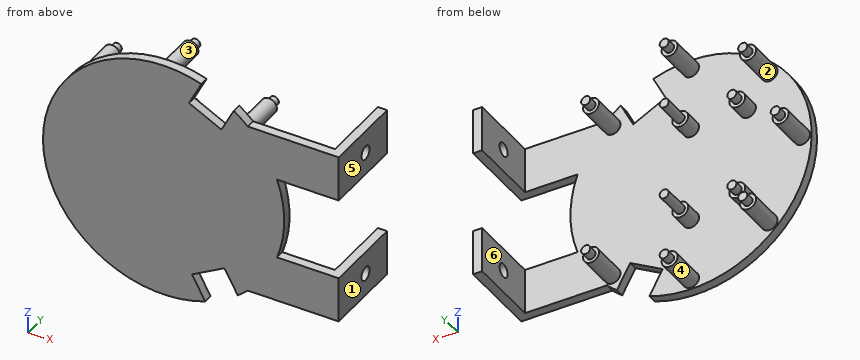
Autodesk Inventor part; units mm, degrees
ref_plane "YZ Plane" through (0, 0, 0) normal (1, 0, 0) x (0, 1, 0)
ref_plane "XZ Plane" through (0, 0, 0) normal (0, 1, 0) x (-1, 0, 0)
ref_plane "XY Plane" through (0, 0, 0) normal (0, 0, 1) x (1, 0, 0)
sketch "Teller" plane through (0, 0, 0) normal (0, 1, 0) x (-1, 0, 0)
  line L0 (-16.2935, -20.8991) -> (-13.3783, -15.6549)
  line L1 (-13.3783, -15.6549) -> (-6.2348, -19.626)
  line L2 (-6.2348, -19.626) -> (-9.15, -24.8702)
  line L3 (-8.2927, 25.1691) -> (-5.5764, 19.8191)
  line L4 (-5.5764, 19.8191) -> (-12.7097, 16.1974)
  line L5 (-12.7097, 16.1974) -> (-15.426, 21.5474)
  arc A0 (-9.15, -24.8702) -> (-8.2927, 25.1691) centre (0, 0) ccw
  line L6 (33, 0) -> (-43, 0) construction
  line L7 (-25, -9) -> (-53, -9) construction
  line L8 (-53, -9) -> (-53, 9) construction
  line L9 (-53, 9) -> (-25, 9) construction
  line L10 (-25, 9) -> (-25, -9) construction
  line L11 (-25, -9) -> (-53, 9) construction
  line L12 (-53, -9) -> (-25, 9) construction
  line L13 (-36.473, -9) -> (-24.9249, -9)
  line L14 (-18.473, -19) -> (-36.473, -19)
  line L15 (-36.473, -19) -> (-36.473, -9)
  line L16 (-36.473, 9) -> (-24.9249, 9)
  line L17 (-18.473, 19) -> (-36.473, 19)
  line L18 (-36.473, 19) -> (-36.473, 9)
  arc A1 (-15.426, 21.5474) -> (-18.473, 19) centre (0, 0) ccw
  arc A2 (-24.9249, 9) -> (-24.9249, -9) centre (0, 0) ccw
  arc A3 (-18.473, -19) -> (-16.2935, -20.8991) centre (0, 0) ccw
  point P0 (-39, 0)
  dimension "d55" = 6
  dimension "d118" = 6
  dimension "d119" = 6
  dimension "d123" = 18
sketch "Dicke Stifte Außen" plane through (0, 0, 0) normal (0, 1, 0) x (-1, 0, 0)
  line L0 (-29.5209, 0) -> (35.6564, 0) construction
  line L1 (0, -38.3382) -> (0, 35) construction
  circle A0 centre (0, -24.4) radius 1.75
  circle A1 centre (0, 0) radius 26.5 construction
  circle A2 centre (17.2534, -17.2534) radius 1.75
  circle A3 centre (24.4, 0) radius 1.75
  circle A4 centre (17.2534, 17.2534) radius 1.75
  circle A5 centre (0, 24.4) radius 1.75
  circle A6 centre (-17.2534, 17.2534) radius 1.75
  circle A7 centre (-24.4, 0) radius 1.75
  circle A8 centre (-17.2534, -17.2534) radius 1.75
  dimension "d83" = 3.5
  dimension "d84" = 53
  dimension "d87" = 360
sketch "Dünne Stifte Außen" plane through (0, 0, 0) normal (0, 1, 0) x (-1, 0, 0)
  circle A0 centre (0, -24.4) radius 1
  circle A1 centre (0, 0) radius 26.5 construction
  circle A2 centre (0, 0) radius 26.5 construction
  circle A3 centre (17.2534, -17.2534) radius 1
  circle A4 centre (24.4, 0) radius 1
  circle A5 centre (17.2534, 17.2534) radius 1
  circle A6 centre (0, 24.4) radius 1
  circle A7 centre (-17.2534, 17.2534) radius 1
  circle A8 centre (-24.4, 0) radius 1
  circle A9 centre (-17.2534, -17.2534) radius 1
  dimension "d90" = 2
  dimension "d91" = 53
  dimension "d92" = 53
  dimension "d95" = 360
sketch "Dicke Stifte Vorn" plane through (0, 0, 0) normal (0, 1, 0) x (-1, 0, 0)
  circle A0 centre (0, 10.5) radius 1.75
  line L0 (-29.5209, 0) -> (35.6564, 0) construction
  circle A1 centre (0, -10.5) radius 1.75
  point P0 (0, 0)
  dimension "d97" = 3.5
sketch "Dicke Stifte Hinten" plane through (0, 0, 0) normal (0, 1, 0) x (-1, 0, 0)
  circle A0 centre (12.5, -10.5) radius 1.75
  line L0 (-29.5209, 0) -> (35.6564, 0) construction
  circle A1 centre (12.5, 10.5) radius 1.75
  point P0 (0, 0)
  dimension "d99" = 3.5
sketch "Dünne Stifte Vorn" plane through (0, 0, 0) normal (0, 1, 0) x (-1, 0, 0)
  circle A0 centre (0, 10.5) radius 1
  line L0 (-29.5209, 0) -> (35.6564, 0) construction
  circle A1 centre (0, -10.5) radius 1
  point P0 (0, 0)
  dimension "d100" = 2
sketch "Dünne Stifte Hinten" plane through (0, 0, 0) normal (0, 1, 0) x (-1, 0, 0)
  circle A0 centre (12.5, -10.5) radius 1
  line L0 (-29.5209, 0) -> (35.6564, 0) construction
  circle A1 centre (12.5, 10.5) radius 1
  point P0 (0, 0)
  dimension "d101" = 2
extrude "Extrusion13" add sketch "Dicke Stifte Außen" along normal blind 8 contours A0 | A2 | A3 | A4 | A5 | A6 | A8
extrude "Extrusion14" add sketch "Dicke Stifte Vorn" along normal blind 4
extrude "Extrusion15" add sketch "Dicke Stifte Hinten" along normal blind 4
extrude "Extrusion16" add sketch "Dünne Stifte Außen" along normal blind 10 contours A0 | A3 | A4 | A5 | A6 | A7 | A9
extrude "Extrusion17" add sketch "Dünne Stifte Vorn" along normal blind 10
extrude "Extrusion18" add sketch "Dünne Stifte Hinten" along normal blind 6
extrude "Extrusion19" add sketch "Teller" against normal blind 2
sketch "Skizze18" plane through (36.473, 0, 19) normal (1, 0, 0) x (0, 0, -1)
  line L0 (0, 16) -> (10, 16)
  line L1 (10, 16) -> (10, -2)
  line L2 (10, -2) -> (0, -2)
  line L3 (0, -2) -> (0, 16)
  line L4 (0, 16) -> (10, -2) construction
  line L5 (10, 16) -> (0, -2) construction
  point P0 (19, 0)
  point P1 (5, 7)
extrude "Extrusion21" add sketch "Skizze18" along normal blind 2
sketch "Skizze19" plane through (36.473, 0, -9) normal (1, 0, 0) x (0, 0, -1)
  line L0 (0, 16) -> (10, 16)
  line L1 (10, 16) -> (10, -2)
  line L2 (10, -2) -> (0, -2)
  line L3 (0, -2) -> (0, 16)
  line L4 (0, 16) -> (10, -2) construction
  line L5 (10, 16) -> (0, -2) construction
  point P0 (-9, 0)
  point P1 (5, 7)
extrude "Extrusion22" add sketch "Skizze19" along normal blind 2
sketch "Skizze20" plane through (36.473, 0, 19) normal (-1, 0, 0) x (0, 0, 1)
  circle A0 centre (-5, 8) radius 1.5
  point P0 (-19, 0)
  dimension "d135" = 3
extrude "Extrusion23" cut sketch "Skizze20" against normal blind 2
sketch "Skizze21" plane through (36.473, 0, -9) normal (-1, 0, 0) x (0, 0, 1)
  circle A0 centre (-5, 8) radius 1.5
  point P0 (9, 0)
  dimension "d138" = 3
extrude "Extrusion24" cut sketch "Skizze21" against normal blind 2
properties part number "Pi Cam Holder"
The listing builds one solid part. Answer for the finished solid, in the listing's coordinates (mm). Face numbers are marked on the shaded views. A direction names the side the tool comes from. Round coordinates to 2 decimals unless told otherwise and drop trailing zeros. Order: outer loops, then holes, each group sorted by start corner. A loop starts at its lowest first (then second) coordinate and runs counter-clockwise, first axis right, second up. Notation, with made-up numbers: M 42.5,-2 L 68.5,-2 A29 cw 68.5,18 Z; hole C 81.5,14.25 d9. An arc over 180 degrees is marked long. Answer in a Markdown table with one row per item. Add a question column.
1) The part is cut by section A-A on z = 14. Determine the outline of the cut face in (x, y), plus the area to 3 significant figures.
2) Consider line 1 along Y through (x, z) = (37.45, 14); line 2 along Y through (x, z) = (7.5, 13); line 3 along X through (y, z) = (10.5, 12.5). Determine where each line is inside the solid, lowest interval first. Write a range as from..to.
3) The part is cut by section C-C on x = -12.5. Determine the outline of the cut face in (y, z).
4) Flat-ended cylindrical pins translate along their axes: pin 1 Ø6 at (x, z) = (16, 11) entering from +Y; pin 2 Ø10 at (x, y) = (17.5, 4) entering from +Z; pin 3 Ø0.6 at (x, z) = (-0.5, 24) entering from +Y. Find the tip coordinate at first contact, or state that the pin passes through.
5) Which of the six approach directions +Z, -Z, +X, -X, +Y, -Y give full straight-line access (tool end or side, diameter ignored) to the marked faces 4, 5 and 6?
6) Determine the mould class of the marked faces 1, 2 and 3 for opening direction X: pulls with the +X half, pulls with the -X half, needs draft (parallel to the pull), parting line crosses it, or undercut.
7) The part is cut by section B-B on y = 4.75. Count the separate pieces of the cut face and the enclosed holes in it, plus the area to 3 significant figures.
8) The part is cut by section D-D on z = 24.4. Determine the outline of the cut face in (x, y), plus the area to 3 significant figures.
Findings below:
| question | item | result |
|---|---|---|
| 1 | outline | M -22.5,-2 L 38.47,-2 L 38.47,6.5 L 36.47,6.5 L 36.47,0 L -22.5,0 Z; M 36.47,9.5 L 38.47,9.5 L 38.47,16 L 36.47,16 Z |
| 1 | area | 148 mm² |
| 2 | line 1 | y = -2..6.5, 9.5..16 |
| 2 | line 2 | y = -2..0 |
| 2 | line 3 | x = 36.47..38.47 |
| 3 | outline | M -2,-23.37 L 0,-23.37 L 0,-12.25 L 4,-12.25 L 4,-11.5 L 6,-11.5 L 6,-9.5 L 4,-9.5 L 4,-8.75 L 0,-8.75 L 0,8.75 L 4,8.75 L 4,9.5 L 6,9.5 L 6,11.5 L 4,11.5 L 4,12.25 L 0,12.25 L 0,23.37 L -2,23.37 Z |
| 4 | pin 1 | stops at y = 0 |
| 4 | pin 2 | stops at z = 21.55 |
| 4 | pin 3 | stops at y = 10 |
| 5 | face 4 | +Y |
| 5 | face 5 | +Z, -Z, +X, +Y, -Y |
| 5 | face 6 | +Z, -Z, +Y |
| 6 | face 1 | pulls with the +X half |
| 6 | face 2 | undercut |
| 6 | face 3 | parting line crosses it |
| 7 | separate pieces | 13 |
| 7 | enclosed holes | 0 |
| 7 | area | 120 mm² |
| 8 | outline | M -10.34,-2 L 7.9,-2 L 7.9,0 L 1.75,0 L 1.75,8 L 1,8 L 1,10 L -1,10 L -1,8 L -1.75,8 L -1.75,0 L -10.34,0 Z |
| 8 | area | 68.5 mm² |
